from build123d import *

# Parameters (mm, degrees)
SKETCH_1_W           = 8.8392
SKETCH_1_H           = 6.2992
EXTRUDE_1_DEPTH      = 1.6256
EXTRUDE_2_DEPTH      = 2.54
SKETCH_3_W           = 5.6261
SKETCH_3_H           = 6.2992
EXTRUDE_3_DEPTH      = 1.6256
SKETCH_4_W           = 6.2992
SKETCH_4_H           = 1.6256
EXTRUDE_4_DEPTH      = 3.2131
HOLE_WIZARD_M2_5_1_D = 2.794
FILLET_1_R           = 0.635
FILLET_2_R           = 1.27


with BuildPart() as part:
    # 草圖1 → 填料-伸長1 (new body)
    with BuildSketch(Plane.XZ.offset(-4.1656)):
        Rectangle(SKETCH_1_W, SKETCH_1_H)
    extrude(amount=-EXTRUDE_1_DEPTH)

    # 草圖2 → 填料-伸長2 (add)
    with BuildSketch(Plane.XZ.offset(-4.1656)):
        with BuildLine():
            Line((-1.2065, 1.474239719), (-1.2065, 3.1496))
            Line((-1.2065, 3.1496), (1.2065, 3.1496))
            Line((1.2065, 3.1496), (1.2065, 1.474239719))
            ThreePointArc((1.2065, 1.474239719), (0, -1.905), (-1.2065, 1.474239719))
        make_face()
    extrude(amount=EXTRUDE_2_DEPTH)

    # 草圖3 → 填料-伸長3 (add)
    with BuildSketch(Plane.XZ.offset(-1.6256)):
        with Locations((-1.60655, 0)):
            Rectangle(SKETCH_3_W, SKETCH_3_H)
    extrude(amount=EXTRUDE_3_DEPTH)

    # 草圖4 → 填料-伸長4 (add)
    with BuildSketch(Plane(origin=(1.2065, 0, 0), x_dir=(0, 0, -1), z_dir=(1, 0, 0))):
        with Locations((0, 0.8128)):
            Rectangle(SKETCH_4_W, SKETCH_4_H)
    extrude(amount=EXTRUDE_4_DEPTH)

    # M2.5 餘隙孔1 (through all)
    with Locations(Plane(origin=(0, 5.7912, 0), x_dir=(1, 0, 0), z_dir=(0, 1, 0))):
        with Locations((0, 0)):
            Hole(HOLE_WIZARD_M2_5_1_D / 2)

    # 圓角1
    fillet_1_edges = [part.edges().sort_by_distance(p)[0] for p in [
        (-1.2065, 2.8956, 3.1496),
        (1.2065, 2.8956, 3.1496),
    ]]
    fillet(fillet_1_edges, radius=FILLET_1_R)

    # 圓角2
    fillet_2_edges = [part.edges().sort_by_distance(p)[0] for p in [
        (-4.4196, 0.8128, 3.1496),
        (-4.4196, 0.8128, -3.1496),
        (4.4196, 0.8128, 3.1496),
        (4.4196, 0.8128, -3.1496),
        (4.4196, 4.9784, -3.1496),
        (-4.4196, 4.9784, -3.1496),
        (-4.4196, 4.9784, 3.1496),
        (4.4196, 4.9784, 3.1496),
    ]]
    fillet(fillet_2_edges, radius=FILLET_2_R)


solid = part.part
CAD build for the part. Positions are in the model's coordinates, mm. A direction names the side the tool comes from. Coordinates: 2 decimals unless noted, no trailing zeros. Write each loop counter-clockwise with the first axis right and the second up, starting at its lowest first coordinate (ties: lowest second). Pieces come first, ordered by that corner, then holes. Notation, with made-up numbers: M 63,-1.75 L 92,-1.75 A9 cw 92,6.25 Z; hole C 29,-29 d2. An arc over 180 degrees is marked long. Answer as a JSON object with one key per item and string values. Group by question number.
1) Saw through at B-B (y = 1.3). Write the cut outline in (x, z).
2) Saw through at C-C (z = -0.75). Write the cut outline in (x, y).
3) Pin check, flat tip, straight feed: pin 1 Ø0.5 at (y, z) = (3.5, 2) entering from -X. Stop position of the tip, or through.
4) Mould opens along Y. For faces 1 (the face through (0.9, 5.791, -1.4)), 2 (the face through (-1.206, 3, 2)), 3 (the face through (0, 3, 3.15)) say: +Y half, -Y half, draft (parallel to the pull), parting line (faces both ways), or undercut.
5) Saw through at A-A (x = 0). Write the cut outline in (y, z) (3 decimals), plus the area to 3 significant figures.
6) Saw through at D-D (z = 2). Write the cut outline in (x, y).
7) Wall check: line 1 (Z direction, x = 0, y = 2.6) (3 decimals); line 2 (Y direction, x = 2.5, z = 0.5); line 3 (Z direction, x = 0, y = 4.6). Give the ranges that are in metal, low to high. Write a range as from..to.
8) Tool access for faces 4 (the face through (1.207, 3, 2)), 5 (the face through (0.065, 2.913, -1.904)), 6 (the face through (4.038, 4.99, -2.787)): list every direction of +Z, -Z, +X, -X, +Y, -Y with a clear straight run to the whole face (end or side of a thin tool).
Values follow:
{
 "1": {"outline": "M -4.42,-1.88 A1.27 ccw -3.15,-3.15 L 3.15,-3.15 A1.27 ccw 4.42,-1.88 L 4.42,1.88 A1.27 ccw 3.15,3.15 L -3.15,3.15 A1.27 ccw -4.42,1.88 Z; hole C 0,0 d2.79"},
 "2": {"outline": "M -4.42,0 L -1.18,0 L -1.18,5.79 L -4.42,5.79 L -4.42,4.17 L -1.75,4.17 L -1.75,1.63 L -4.42,1.63 Z; M 1.18,0 L 4.42,0 L 4.42,1.63 L 1.75,1.63 L 1.75,4.17 L 4.42,4.17 L 4.42,5.79 L 1.18,5.79 Z"},
 "3": {"pin 1": "stops at x = -1.21"},
 "4": {"face 1": "+Y half", "face 2": "undercut", "face 3": "draft"},
 "5": {"outline": "M 0,-3.15 L 1.626,-3.15 L 1.626,-1.905 L 4.166,-1.905 L 4.166,-3.15 L 5.791,-3.15 L 5.791,-1.397 L 0,-1.397 Z; M 0,1.397 L 5.791,1.397 L 5.791,3.15 L 0,3.15 Z", "area": "17.1 mm2"},
 "6": {"outline": "M -4.41,0 L 4.41,0 L 4.41,1.63 L 1.21,1.63 L 1.21,4.17 L 4.41,4.17 L 4.41,5.79 L -4.41,5.79 L -4.41,4.17 L -1.21,4.17 L -1.21,1.63 L -4.41,1.63 Z"},
 "7": {"line 1": "z = -1.905..-1.397, 1.397..3.15", "line 2": "y = 0..1.63, 4.17..5.79", "line 3": "z = -3.15..-1.4, 1.4..3.15"},
 "8": {"face 4": "+Z, +X", "face 5": "none", "face 6": "-Z, +X, +Y, -Y"}
}
